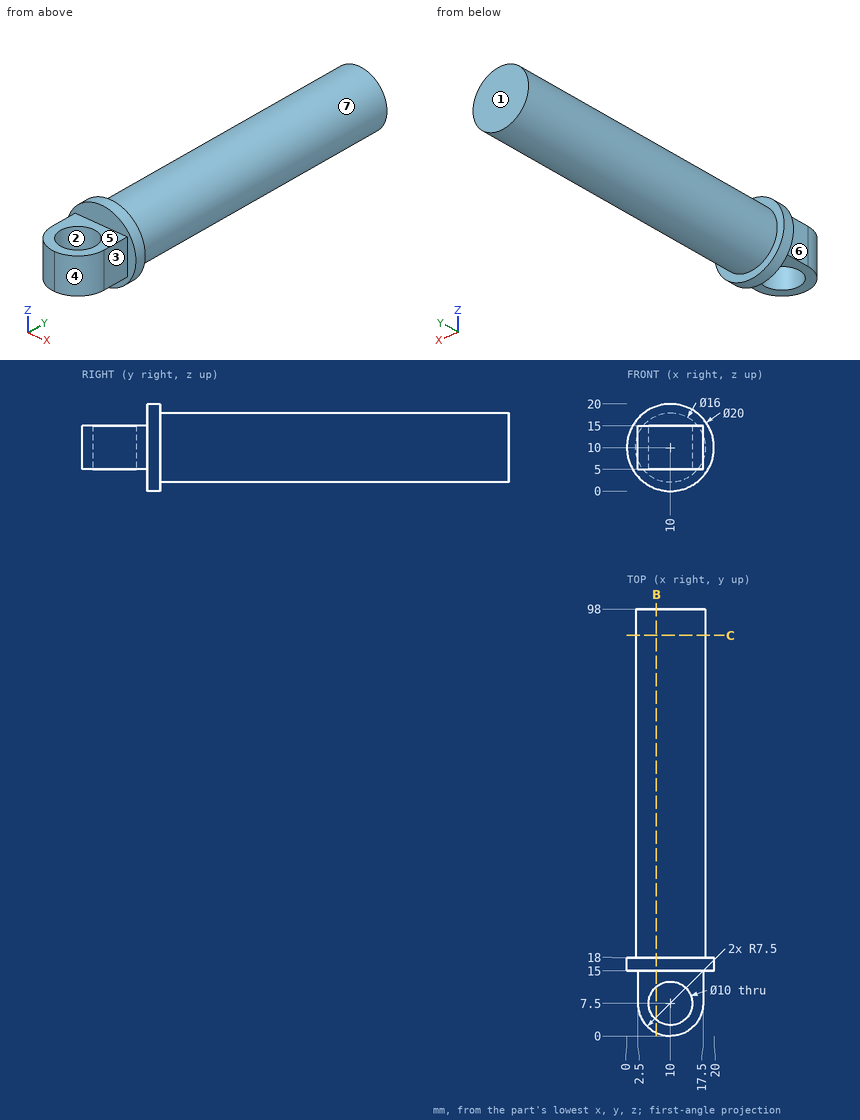
The figure shows three views and two pictorial views of one solid part (mm, origin at its lowest corner). Answer the questions. A direction names the side the tool comes from. Give positions to 0.01 mm unless a question says otherwise; leave off trailing zeros. Loops run counter-clockwise (first coordinate to the right, second up) from the corner with the lowest first, then second, coordinate; pieces in that order, holes last. Notation, with made-up numbers: (-22, 84.5) -> (11, 84.5) arc R16 cw to (11, 105.5) -> close; hole circle Ø10 at (58, -8). An arc over 180 degrees is marked (long way). Put each result on its own line as item: value. Start each with the question number.
Item 1: Find the intervals of material crossed by L1, parallel to Y at x = 10, z = 9.25; L2, parallel to Z at x = 8.5, y = 12.5; L3, parallel to Y at x = 12.25, z = 12.75 (1 decimal), in increasing order. Write a range as [from, to].
Item 2: The part is cut by section B-B (x = 6.75). Give the vertices of the cut face in (y, z).
Item 3: Which of the six approach directions +Z, -Z, +X, -X, +Y, -Y give full straight-line access (tool end or side, diameter ignored) to the marked faces 5, 6 and 7?
Item 4: The part is cut by section C-C (y = 92). Give the vertices of the cut face in (x, z), then the cut area to 3 significant figures.
Item 5: Each of these flat-tipped pins is pushed along its axis until it touches: P1, Ø4, axis at x = 14.5, z = 12.5, coming from the -Y side; P2, Ø1, axis at x = 6, y = 57, coming from the -Z side; P3, Ø11.5, axis at x = 10, y = 7.5, coming from the +Z side. Where does it stop, or does it pass through?
Item 6: The mould has two halves that part along Y. Classify the marked faces 1, 2, 3 and 4: released by +Y, released by -Y, zero draft, split by the parting line, or undercut.
Answers below:
1. L1: [0, 2.5], [12.5, 98]
1. L2: [5, 15]
1. L3: [0.3, 3], [12, 98]
2. outline: (0.74, 5) -> (3.7, 5) -> (3.7, 15) -> (0.74, 15) -> close; (11.3, 5) -> (15, 5) -> (15, 0.54) -> (18, 0.54) -> (18, 2.69) -> (98, 2.69) -> (98, 17.31) -> (18, 17.31) -> (18, 19.46) -> (15, 19.46) -> (15, 15) -> (11.3, 15) -> close
3. face 5: +Z, +X, -X, -Y
3. face 6: +Z, -Z, -X, -Y
3. face 7: +Y
4. outline: circle Ø16 at (10, 10)
4. area: 201 mm2
5. P1: y = 0.43
5. P2: z = 2.81
5. P3: z = 15
6. face 1: released by +Y
6. face 2: undercut
6. face 3: zero draft
6. face 4: released by -Y
